from build123d import *

# Parameters (mm, degrees)
PAD_DEPTH   = 40
FILLET_R    = 2
FILLET001_R = 1


with BuildPart() as part:
    # Sketch → Pad (new body)
    with BuildSketch(Plane.XY):
        Polygon((-15.75, 28), (15.75, 28), (15.75, 20), (25.75, 20), (20.5, -20), (12.5, -20), (12.5, -28), (-12.5, -28), (-12.5, -20), (-20.5, -20), (-25.75, 20), (-15.75, 20), align=None)
        with BuildLine():
            ThreePointArc((12.5, 7.5), (0, 20), (-12.5, 7.5))
            Line((-12.5, 7.5), (-12.5, -7.5))
            ThreePointArc((-12.5, -7.5), (0, -20), (12.5, -7.5))
            Line((12.5, 7.5), (12.5, -7.5))
        make_face(mode=Mode.SUBTRACT)
    extrude(amount=PAD_DEPTH)

    # Fillet
    fillet_edges = [part.edges().sort_by_distance(p)[0] for p in [
        (25.75, 20, 20),
        (15.75, 28, 20),
        (-15.75, 28, 20),
        (-25.75, 20, 20),
        (-20.5, -20, 20),
        (-12.5, -28, 20),
        (12.5, -28, 20),
        (20.5, -20, 20),
    ]]
    fillet(fillet_edges, radius=FILLET_R)

    # Fillet001
    fillet001_edges = [part.edges().sort_by_distance(p)[0] for p in [
        (15.75, 20, 20),
        (-15.75, 20, 20),
        (12.5, -20, 20),
        (-12.5, -20, 20),
    ]]
    fillet(fillet001_edges, radius=FILLET001_R)


solid = part.part
Work out the finished part from the listing and answer in its coordinate system (mm). A direction names the side the tool comes from. Give positions to 0.01 mm unless a question says otherwise; leave off trailing zeros. Loops run counter-clockwise (first coordinate to the right, second up) from the corner with the lowest first, then second, coordinate; pieces in that order, holes last. Notation, with made-up numbers: (26, 73) - (45, 73) arc R16 ccw to (45, 86) - close; hole circle Ø1 at (33, -8). An arc over 180 degrees is marked (long way). Answer in a Markdown table with one row per item. Add a question column.
Q1. A tool of negligible diameter and unlimited length cuts with its end or side. For faces 5 (the flat face through (-16, -20, 20)), 6 (the flat face through (15.75, 24, 20)), 7 (the flat face through (16, -20, 20)), 8 (the flat face through (-12.5, 0, 20)), from which of +Z, -Z, +X, -X, +Y, -Y can it reach the whole face along a straight path? Write none if from no direction.
Q2. The part is cut by section A-A (x = -0.5). Determine the outline of the cut face in (y, z), and give its area (3 significant figures).
Q3. Each of these flat-tipped pins is pushed along its axis until it touches: P1, Ø2, axis at x = 20.5, z = 28, coming from the +Y side; P2, Ø6, axis at y = 10.5, z = 30.5, coming from the -X side; P3, Ø4.5, axis at y = 0, z = 27.5, coming from the -X side. Where does it stop, or does it pass through?
Q4. Determine the mould class of faces 1 (the flat face through (-15.75, 23, 20)), 2 (the flat face through (-23.06, -0.51, 19.72)), 3 (the flat face through (20, 20, 20)), 4 (the cylindrical face through (0, 20, 20)) for opening direction Y: released by +Y, released by -Y, zero draft, split by the parting line, or undercut.
Q5. Consider line 1 along X through (y, z) = (-23.5, 34); line 2 along X through (y, z) = (-14.5, 31); line 3 along X through (y, z) = (0.5, 25). Determine where each line is inside the solid, lowest interval first.
Q6. The part is cut by section C-C (y = 2). Determine the outline of the cut face in (x, z).
Q7. The part is cut by section D-D (x = -18). Determine the outline of the cut face in (y, z).
Q8. The part is cut by section B-B (z = 33.5). Determine the outline of the cut face in (x, y).
Solution:
| question | item | result |
|---|---|---|
| 1 | face 5 | +Z, -Z, -X, -Y |
| 1 | face 6 | +Z, -Z, +X, +Y |
| 1 | face 7 | +Z, -Z, +X, -Y |
| 1 | face 8 | +Z, -Z |
| 2 | outline | (-28, 0) - (-19.99, 0) - (-19.99, 40) - (-28, 40) - close; (19.99, 0) - (28, 0) - (28, 40) - (19.99, 40) - close |
| 2 | area | 641 mm² |
| 3 | P1 | stops at y = 20 |
| 3 | P2 | stops at x = -24.9 |
| 3 | P3 | stops at x = -23.42 |
| 4 | face 1 | zero draft |
| 4 | face 2 | released by -Y |
| 4 | face 3 | released by +Y |
| 4 | face 4 | undercut |
| 5 | line 1 | x = -12.5 to 12.5 |
| 5 | line 2 | x = -21.22 to -10.36, 10.36 to 21.22 |
| 5 | line 3 | x = -23.19 to -12.5, 12.5 to 23.19 |
| 6 | outline | (-23.39, 0) - (-12.5, 0) - (-12.5, 40) - (-23.39, 40) - close; (12.5, 0) - (23.39, 0) - (23.39, 40) - (12.5, 40) - close |
| 7 | outline | (-20, 0) - (20, 0) - (20, 40) - (-20, 40) - close |
| 8 | outline | (-25.45, 17.74) - (-20.73, -18.26) arc R2 ccw to (-18.75, -20) - (-13.5, -20) arc R1 cw to (-12.5, -21) - (-12.5, -26) arc R2 ccw to (-10.5, -28) - (10.5, -28) arc R2 ccw to (12.5, -26) - (12.5, -21) arc R1 cw to (13.5, -20) - (18.75, -20) arc R2 ccw to (20.73, -18.26) - (25.45, 17.74) arc R2 ccw to (23.47, 20) - (16.75, 20) arc R1 cw to (15.75, 21) - (15.75, 26) arc R2 ccw to (13.75, 28) - (-13.75, 28) arc R2 ccw to (-15.75, 26) - (-15.75, 21) arc R1 cw to (-16.75, 20) - (-23.47, 20) arc R2 ccw to start; hole (-12.5, -7.5) arc R12.5 ccw to (12.5, -7.5) - (12.5, 7.5) arc R12.5 ccw to (-12.5, 7.5) - close |
